Geometry: final body of the model. Coordinates: model frame, mm. Face numbers are marked on the shaded views. A direction names the side the tool comes from. Coordinates: 2 decimals unless noted, no trailing zeros. Order: outer loops, then holes, each group sorted by start corner. A loop starts at its lowest first (then second) coordinate and runs counter-clockwise, first axis right, second up. Notation, with made-up numbers: (-31, -35.5) -> (0, -35.5) arc R30 ccw to (0, -13.5) -> close; hole circle Ø8 at (14.5, -40). An arc over 180 degrees is marked (long way). Answer in a Markdown table with one row per item. Add a question column.
1) Section query D-D on x = 2.25. Return the cut outline in (y, z) (3 decimals), then the cut area to 3 significant figures.
2) Contact query for flat-ended pins moving along their axis: P1, Ø1.1, axis at x = 0.5, z = 3.5, coming from the +Y side (3 decimals); P2, Ø0.8, axis at x = 0, z = 4, coming from the -Y side (3 decimals); P3, Ø1.5, axis at y = -1.5, z = 5, coming from the -X side. Output: stop coordinate, or through.
3) Ray query, line 1 (Y direction, x = -0.75, z = 2.75) (3 decimals); line 2 (X direction, y = 2.75, z = 6.5); line 3 (Z direction, x = 1.5, y = -5.5). Return the intervals inside material, ascending. Write a range as from..to.
4) Section query A-A on x = -0.5. Return the cut outline in (y, z) (3 decimals), then the cut area to 3 significant figures.
5) Section query B-B on z = 5.25. Return the cut outline in (x, y) (3 decimals), then the cut area to 3 significant figures.
6) Set-up query: the marked faces 1, 2 and 3. Return all of +Z, -Z, +X, -X, +Y, -Y with unobstructed straight access to the full face (end or side cutting, diameter ignored); none if empty.
7) Section query C-C on y = -2.5. Return the cut outline in (x, z), then the cut area to 3 significant figures.
8) Pull-direction query (X, two-part tool) for the marked faces 4, 5 and 6; classes: +X half, -X half, draft (parallel to the pull), parting line (faces both ways), or undercut.
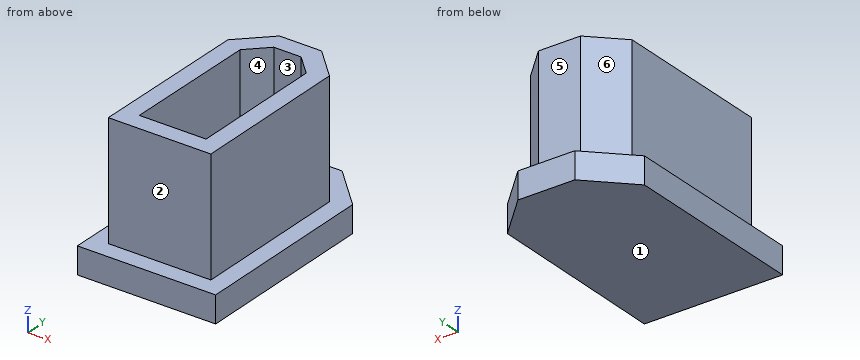
```python
from build123d import *

# Parameters (mm, degrees)
F1_DEPTH = 8
F2_DEPTH = 1.5


with BuildPart() as f1:
    # F0 (on Top) → F1 (new body)
    with BuildSketch(Plane.XY):
        Polygon((-1.180977, 5.375), (-2.849841, 3.706136), (-2.878119, -5.375), (2.878119, -5.375), (2.849841, 3.706136), (1.180977, 5.375), align=None)
        Polygon((1.85113, 3.290633), (1.875, -4.375), (-1.875, -4.375), (-1.85113, 3.290633), (-0.766763, 4.375), (0.766763, 4.375), align=None, mode=Mode.SUBTRACT)
    extrude(amount=F1_DEPTH)

    # F0 (on Top) → F2 (join)
    with BuildSketch(Plane.XY):
        Polygon((-1.59519, 6.375), (-3.848552, 4.121638), (-3.881237, -6.375), (3.881237, -6.375), (3.848552, 4.121638), (1.59519, 6.375), align=None)
        Polygon((-2.878119, -5.375), (-2.849841, 3.706136), (-1.180977, 5.375), (1.180977, 5.375), (2.849841, 3.706136), (2.878119, -5.375), align=None, mode=Mode.SUBTRACT)
        Polygon((-1.875, -4.375), (1.875, -4.375), (1.85113, 3.290633), (1.85113, 1.757106), (0.766763, 0.672739), (-0.766763, 0.672739), (-1.85113, 1.757106), (-1.85113, 3.290633), align=None)
        Polygon((1.85113, 1.757106), (1.85113, 3.290633), (0.766763, 4.375), (-0.766763, 4.375), (-1.85113, 3.290633), (-1.85113, 1.757106), (-0.766763, 0.672739), (0.766763, 0.672739), align=None)
    extrude(amount=F2_DEPTH)


solid = f1.part
```
Result:
| question | item | result |
|---|---|---|
| 1 | outline | (-6.375, 0) -> (5.72, 0) -> (5.72, 1.5) -> (4.306, 1.5) -> (4.306, 8) -> (-5.375, 8) -> (-5.375, 1.5) -> (-6.375, 1.5) -> close |
| 1 | area | 81.1 mm2 |
| 2 | P1 | y = 5.375 |
| 2 | P2 | y = -5.375 |
| 2 | P3 | x = -2.87 |
| 3 | line 1 | -5.375..-4.375, 4.375..5.375 |
| 3 | line 2 | -2.85..-1.85, 1.85..2.85 |
| 3 | line 3 | 0..1.5 |
| 4 | outline | (-6.375, 0) -> (6.375, 0) -> (6.375, 1.5) -> (5.375, 1.5) -> (5.375, 8) -> (4.375, 8) -> (4.375, 1.5) -> (-4.375, 1.5) -> (-4.375, 8) -> (-5.375, 8) -> (-5.375, 1.5) -> (-6.375, 1.5) -> close |
| 4 | area | 32.1 mm2 |
| 5 | outline | (-2.878, -5.375) -> (2.878, -5.375) -> (2.85, 3.706) -> (1.181, 5.375) -> (-1.181, 5.375) -> (-2.85, 3.706) -> close; hole (-1.875, -4.375) -> (1.875, -4.375) -> (1.851, 3.291) -> (0.767, 4.375) -> (-0.767, 4.375) -> (-1.851, 3.291) -> close |
| 5 | area | 27.3 mm2 |
| 6 | face 1 | -Z, +X, -X, +Y, -Y |
| 6 | face 2 | +Z, +X, -X, -Y |
| 6 | face 3 | +Z |
| 7 | outline | (-3.87, 0) -> (3.87, 0) -> (3.87, 1.5) -> (2.87, 1.5) -> (2.87, 8) -> (1.87, 8) -> (1.87, 1.5) -> (-1.87, 1.5) -> (-1.87, 8) -> (-2.87, 8) -> (-2.87, 1.5) -> (-3.87, 1.5) -> close |
| 7 | area | 24.6 mm2 |
| 8 | face 4 | undercut |
| 8 | face 5 | draft |
| 8 | face 6 | -X half |
